Geometry: final body of the model. Coordinates: model frame, mm. A direction names the side the tool comes from. Give positions to 0.01 mm unless a question says otherwise; leave off trailing zeros. Write each loop counter-clockwise with the first axis right and the second up, starting at its lowest first coordinate (ties: lowest second). Pieces come first, ordered by that corner, then holes. Notation, with made-up numbers: (64, 59) -> (102, 59) arc R32 ccw to (102, 93) -> close; hole circle Ø8 at (1, 45). An arc over 180 degrees is marked (long way). Answer in a Markdown table with one row per item. Add a question column.
Item 1: First-contact query: P1, Ø5, axis at y = 23, z = 1, coming from the +X side; P2, Ø2, axis at x = -13.5, z = 3, coming from the -Y side; P3, Ø2, axis at x = 14.22, z = 0, coming from the +Y side; P4, Ø3, axis at x = -1.5, z = -4, coming from the +Y side. Flat tips, straight axial feed; report the tip coordinate or a pass-through.
Item 2: Section query C-C on y = 21. Output: boundary loops of the cut face in (x, z).
Item 3: Section query B-B on x = 14.22. Output: boundary loops of the cut face in (y, z).
Item 4: Section query A-A on x = 5.65. Output: boundary loops of the cut face in (y, z).
Item 5: Access query for faces 1 (the flat face through (-12.6, 20.35, -0.1)), 2 (the flat face through (12.6, 19, -0.1)), 3 (the cylindrical face through (3.666, 31.109, 1.521)). Directions: +Z, -Z, +X, -X, +Y, -Y. A direction counts if a zero-diameter tool reaches every point of the face in a straight line with its end or side. Return the directions, or none.
Item 6: Material intervals for probe 1 along X at (y, z) = (21.5, 0); probe 2 along Z at (x, y) = (-12, 21); probe 3 along Y at (x, z) = (-14, -4), sorted ascending. Write a range as from..to.
Item 7: Section query D-D on y = 17.5. Output: boundary loops of the cut face in (x, z) (3 decimals).
```python
from build123d import *

# Parameters (mm, degrees)
SKETCH2_W           = 22.83
SKETCH2_H           = 12.1
BOSS_EXTRUDE1_DEPTH = 19
SKETCH3_W           = 31.28
SKETCH3_H           = 12.1
BOSS_EXTRUDE2_DEPTH = 5.6
CUT_EXTRUDE1_DEPTH  = 13.1
SKETCH6_W           = 4.22
SKETCH6_H           = 8.48
CUT_EXTRUDE2_DEPTH  = 4.25
CUT_EXTRUDE3_REACH  = 22.35
SKETCH7_R           = 1.4
SKETCH8_R           = 5.77
SKETCH8_R_2         = 3.085
BOSS_EXTRUDE3_DEPTH = 3.73
SKETCH9_R           = 4.59
SKETCH9_R_2         = 1.61
BOSS_EXTRUDE4_DEPTH = 1.3
SKETCH10_R          = 2.5
BOSS_EXTRUDE5_DEPTH = 3
SKETCH12_R          = 0.89
CUT_EXTRUDE4_DEPTH  = 14


with BuildPart() as part:
    # Sketch2 → Boss-Extrude1 (new body)
    with BuildSketch(Plane(origin=(0, 0, 0), x_dir=(1, 0, 0), z_dir=(0, 1, 0))):
        Rectangle(SKETCH2_W, SKETCH2_H)
    extrude(amount=BOSS_EXTRUDE1_DEPTH)

    # Sketch3 → Boss-Extrude2 (add)
    with BuildSketch(Plane(origin=(0, 19, 0), x_dir=(1, 0, 0), z_dir=(0, 1, 0))):
        Rectangle(SKETCH3_W, SKETCH3_H)
    extrude(amount=BOSS_EXTRUDE2_DEPTH)

    # Sketch5 → Cut-Extrude1 (cut, through all)
    with BuildSketch(Plane.XY.offset(6.05)):
        Polygon((-15.64, 20.35), (-11.42, 24.6), (-15.64, 24.6), align=None)
        Polygon((15.64, 24.6), (15.64, 20.35), (11.42, 24.6), align=None)
    extrude(amount=-CUT_EXTRUDE1_DEPTH, mode=Mode.SUBTRACT)

    # Sketch6 → Cut-Extrude2 (cut)
    with BuildSketch(Plane(origin=(0, 24.6, 0), x_dir=(1, 0, 0), z_dir=(0, 1, 0))):
        with Locations((13.53, 0)):
            Rectangle(SKETCH6_W, SKETCH6_H)
        with Locations((-13.53, 0)):
            Rectangle(SKETCH6_W, SKETCH6_H)
    extrude(amount=-CUT_EXTRUDE2_DEPTH, mode=Mode.SUBTRACT)

    # Sketch7 → Cut-Extrude3 (cut, up to next)
    with BuildSketch(Plane(origin=(0, 20.35, 0), x_dir=(1, 0, 0), z_dir=(0, 1, 0)), mode=Mode.PRIVATE) as cut_extrude3_sk1:
        with Locations((14.22, 0)):
            Circle(SKETCH7_R)
    cut_extrude3_tool1 = extrude(cut_extrude3_sk1.sketch, amount=-CUT_EXTRUDE3_REACH, mode=Mode.PRIVATE) & part.part
    add(cut_extrude3_tool1.solids().sort_by_distance((14.22, 20.35, 0))[0], mode=Mode.SUBTRACT)
    # Sketch7 → Cut-Extrude3 (cut, up to next)
    with BuildSketch(Plane(origin=(0, 20.35, 0), x_dir=(1, 0, 0), z_dir=(0, 1, 0)), mode=Mode.PRIVATE) as cut_extrude3_sk2:
        with Locations((-14.22, 0)):
            Circle(SKETCH7_R)
    cut_extrude3_tool2 = extrude(cut_extrude3_sk2.sketch, amount=-CUT_EXTRUDE3_REACH, mode=Mode.PRIVATE) & part.part
    add(cut_extrude3_tool2.solids().sort_by_distance((-14.22, 20.35, 0))[0], mode=Mode.SUBTRACT)

    # Sketch8 → Boss-Extrude3 (add)
    with BuildSketch(Plane(origin=(0, 24.6, 0), x_dir=(1, 0, 0), z_dir=(0, 1, 0))):
        with Locations((5.65, 0)):
            Circle(SKETCH8_R)
        with Locations((-0.305, 0)):
            Circle(SKETCH8_R_2)
    extrude(amount=BOSS_EXTRUDE3_DEPTH)

    # Sketch9 → Boss-Extrude4 (add)
    with BuildSketch(Plane(origin=(0, 28.33, 0), x_dir=(1, 0, 0), z_dir=(0, 1, 0))):
        with Locations((5.65, 0)):
            Circle(SKETCH9_R)
        with Locations((-0.305, 0)):
            Circle(SKETCH9_R_2)
    extrude(amount=BOSS_EXTRUDE4_DEPTH)

    # Sketch10 → Boss-Extrude5 (add)
    with BuildSketch(Plane(origin=(0, 29.63, 0), x_dir=(1, 0, 0), z_dir=(0, 1, 0))):
        with Locations((5.65, 0)):
            Circle(SKETCH10_R)
    extrude(amount=BOSS_EXTRUDE5_DEPTH)

    # Sketch12 → Cut-Extrude4 (cut)
    with BuildSketch(Plane(origin=(0, 32.63, 0), x_dir=(1, 0, 0), z_dir=(0, 1, 0))):
        with Locations((5.65, 0)):
            Circle(SKETCH12_R)
    extrude(amount=-CUT_EXTRUDE4_DEPTH, mode=Mode.SUBTRACT)


solid = part.part
```
Findings below:
| question | item | result |
|---|---|---|
| 1 | P1 | stops at x = 11.42 |
| 1 | P2 | stops at y = 19 |
| 1 | P3 | passes through |
| 1 | P4 | stops at y = 28.33 |
| 2 | outline | (-14.99, -6.05) -> (14.99, -6.05) -> (14.99, -4.24) -> (11.42, -4.24) -> (11.42, 4.24) -> (14.99, 4.24) -> (14.99, 6.05) -> (-14.99, 6.05) -> (-14.99, 4.24) -> (-11.42, 4.24) -> (-11.42, -4.24) -> (-14.99, -4.24) -> close; hole circle Ø1.78 at (5.65, 0) |
| 3 | outline | (19, -6.05) -> (21.78, -6.05) -> (21.78, -4.24) -> (20.35, -4.24) -> (20.35, -1.4) -> (19, -1.4) -> close; (19, 1.4) -> (20.35, 1.4) -> (20.35, 4.24) -> (21.78, 4.24) -> (21.78, 6.05) -> (19, 6.05) -> close |
| 4 | outline | (0, -6.05) -> (24.6, -6.05) -> (24.6, -5.77) -> (28.33, -5.77) -> (28.33, -4.59) -> (29.63, -4.59) -> (29.63, -2.5) -> (32.63, -2.5) -> (32.63, -0.89) -> (18.63, -0.89) -> (18.63, 0.89) -> (32.63, 0.89) -> (32.63, 2.5) -> (29.63, 2.5) -> (29.63, 4.59) -> (28.33, 4.59) -> (28.33, 5.77) -> (24.6, 5.77) -> (24.6, 6.05) -> (0, 6.05) -> close |
| 5 | face 1 | -X, +Y |
| 5 | face 2 | +Z, -Z, +X, -Y |
| 5 | face 3 | +Y |
| 6 | probe 1 | x = -11.42..4.76, 6.54..11.42 |
| 6 | probe 2 | z = -6.05..-4.24, 4.24..6.05 |
| 6 | probe 3 | y = 19..20.35 |
| 7 | outline | (-11.415, -6.05) -> (11.415, -6.05) -> (11.415, 6.05) -> (-11.415, 6.05) -> close |
